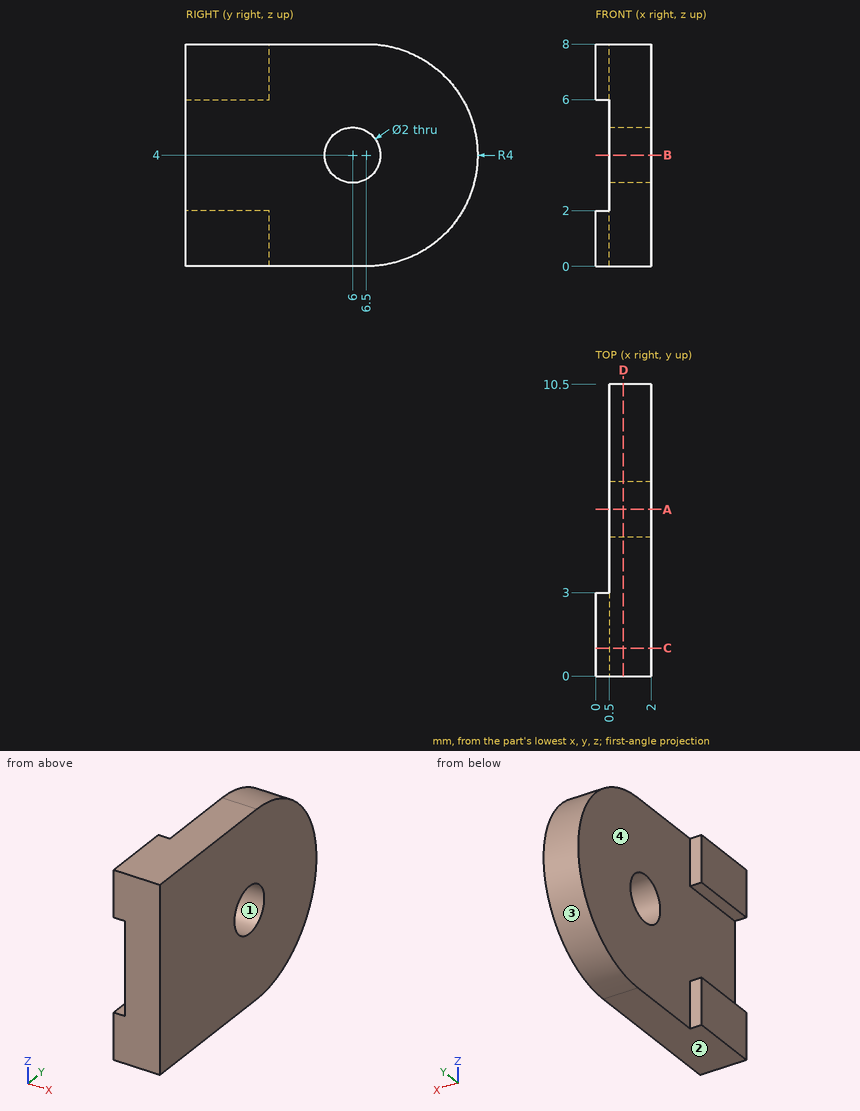
Here's the drawing with two shaded views (mm, measured from the low corner). I have some questions. Give positions to 0.01 mm unless a question says otherwise; leave off trailing zeros. Order: outer loops, then holes, each group sorted by start corner. A loop starts at its lowest first (then second) coordinate and runs counter-clockwise, first axis right, second up. Notation, with made-up numbers: M 77.5,2 L 116.5,2 A17 cw 116.5,28 Z; hole C 25.25,54 d4. An arc over 180 degrees is marked long. Answer as a JSON object with one key per item and string values. Group by question number.
1) I'm going to push flat-ended pins straight in: pin 1 Ø2.5 at (y, z) = (6, 4) entering from -X; pin 2 Ø0.6 at (x, z) = (0, 6.5) entering from +Y. Where does each tip first touch, or does it pass through?
2) Suppose I cut it at B-B, the plane z = 4. Write out the boundary of the cut face in (x, y), plus the area to 4 significant figures.
3) Suppose I cut it at C-C, the plane y = 1. Write out the boundary of the cut face in (x, z), plus the area to 3 significant figures.
4) Suppose I cut it at D-D, the plane x = 1. Write out the boundary of the cut face in (y, z), plus the area to 3 significant figures.
5) Please list where these lines run through material, in increasing order: L1, parallel to Y at x = 1.5, z = 4; L2, parallel to X at y = 3.5, z = 2; L3, parallel to Z at x = 1.4, y = 6.25. Write a range as [from, to].
6) We'd pull the mould along Z, two halves only. Please class the marked faces 1, 2, 3 and 4: pulls with the +Z half, pulls with the -Z half, needs draft (parallel to the pull), parting line crosses it, or undercut.
7) Suppose I cut it at A-A, the plane y = 6. Write out the boundary of the cut face in (x, z), plus the area to 3 significant figures.
Results found:
{
 "1": {"pin 1": "x = 0.5", "pin 2": "y = 3"},
 "2": {"outline": "M 0.5,0 L 2,0 L 2,5 L 0.5,5 Z; M 0.5,7 L 2,7 L 2,10.5 L 0.5,10.5 Z", "area": "12.75 mm²"},
 "3": {"outline": "M 0,0 L 2,0 L 2,8 L 0,8 L 0,6 L 0.5,6 L 0.5,2 L 0,2 Z", "area": "14.0 mm²"},
 "4": {"outline": "M 0,0 L 6.5,0 A4 ccw 6.5,8 L 0,8 Z; hole C 6,4 d2", "area": "74.0 mm²"},
 "5": {"L1": "[0, 5], [7, 10.5]", "L2": "[0.5, 2]", "L3": "[0, 3.03], [4.97, 8]"},
 "6": {"face 1": "undercut", "face 2": "pulls with the -Z half", "face 3": "parting line crosses it", "face 4": "undercut"},
 "7": {"outline": "M 0.5,0 L 2,0 L 2,3 L 0.5,3 Z; M 0.5,5 L 2,5 L 2,8 L 0.5,8 Z", "area": "9.00 mm²"}
}
